Autodesk Inventor part; units mm, degrees
ref_plane "plane_support" through (-5.5, -8, -3) normal (0, -1, 0) x (1, 0, 0)
ref_plane "YZ Plane" through (0, 0, 0) normal (1, 0, 0) x (0, 1, 0)
ref_plane "XZ Plane" through (0, 0, 0) normal (0, 1, 0) x (-1, 0, 0)
sketch "Sketch14" plane through (0, 0, 0) normal (1, 0, 0) x (0, 1, 0)
  line L0 (-13.2, 0) -> (16.2, 0)
  line L1 (0, -4.2) -> (0, 4.2)
  line L2 (9, -3) -> (-9, -3)
  line L3 (-9, -3) -> (-9, 3)
  line L4 (-9, 3) -> (9, 3)
  line L5 (9, 3) -> (9, -3) construction
  line L6 (9, -3) -> (-9, 3) construction
  line L7 (-9, -3) -> (9, 3) construction
  line L8 (5.5, 3) -> (5.5, -3) construction
  line L9 (-6.5, 3) -> (-6.5, -3) construction
  arc A0 (9, -3) -> (9, 3) centre (9, 0) ccw
  circle A1 centre (9, 0) radius 1.25
  circle A2 centre (9, 0) radius 3 construction
  line L10 (6, 3) -> (6, -3) construction
  line L11 (12, -3) -> (9, -3)
  line L12 (9, -3) -> (9, 3)
  line L13 (9, 3) -> (12, 3)
  line L14 (12, 3) -> (12, -3)
  line L15 (12, -3) -> (9, 3) construction
  line L16 (9, -3) -> (12, 3) construction
  point P0 (0, 0)
  point P1 (0, 0)
  point P2 (10.5, 0)
  dimension "d72" = 6
  dimension "d73" = 12
  dimension "d74" = 2.5
  dimension "d75" = 2.5
  dimension "d76" = 0.5
extrude "ext_main" add sketch "Sketch14" along normal mid plane 11
sketch "sk_channel_nut" plane through (-5.5, -9, -3) normal (0, -1, 0) x (1, 0, 0)
  line L0 (-2.2, 3) -> (13.2, 3)
  line L1 (5.5, -1.8497) -> (5.5, 7.8497)
  circle A0 centre (5.5, 3) radius 2
  line L2 (5.5, 6.4641) -> (2.5, 4.7321)
  line L3 (2.5, 4.7321) -> (2.5, 1.2679)
  line L4 (2.5, 1.2679) -> (5.5, -0.4641)
  line L5 (5.5, -0.4641) -> (8.5, 1.2679)
  line L6 (8.5, 1.2679) -> (8.5, 4.7321)
  line L7 (8.5, 4.7321) -> (5.5, 6.4641)
  circle A1 centre (1.5, 3) radius 1
  circle A2 centre (9.5, 3) radius 1
  line L8 (1.5, 4) -> (2.5, 4)
  line L9 (1.5, 2) -> (2.5, 2)
  line L10 (9.5, 4) -> (8.5, 4)
  line L11 (9.5, 2) -> (8.5, 2)
  line L12 (11, 0) -> (0, 0)
  line L13 (11, 6) -> (0, 6)
  line L14 (0, 0) -> (0, 6)
  line L15 (3.4, 6) -> (3.4, 5.2517)
  line L16 (3.4456, 0.722) -> (3.4456, 0)
  line L17 (7.5544, 0.722) -> (7.5544, 0)
  line L18 (7.6, 6) -> (7.6, 5.2517)
  point P0 (5.5, 3)
  point P1 (2.5, 3)
  dimension "d85" = 4
  dimension "d86" = 120
  dimension "d87" = 6
  dimension "d88" = 2
  dimension "d95" = 4.2
extrude "ext_cut_bottomscrews" cut sketch "sk_channel_nut" against normal blind 8 contours A2 L0 | A2 L11 L6 | L6 L10 A2 | L0 A2
extrude "ext_cut_bottom_nut" cut sketch "sk_channel_nut" against normal blind 2 contours L3 L2 L13 L1 A0 L0 | L0 A0 L1 L12 L4 L3 | L16 L4 L12 | L13 L2 L15 | A0 L1 L0 | L0 L1 A0 | L12 L1 L4 | L2 L1 L13 | L1 A0 L0 | L0 A0 L1 | L1 L13 L7 L6 L0 A0 | A0 L0 L6 L5 L12 L1 | L1 L12 L5 | L7 L13 L1 | L5 L17 L12 | L13 L18 L7
sketch "Sketch21" plane through (-5.5, 12, 3) normal (0, 0, 1) x (1, 0, 0)
  line L0 (11, 0) -> (11, -21)
  line L1 (0, 0) -> (11, 0)
  line L2 (0, -21) -> (0, 0)
  line L3 (3.4, -19) -> (7.6, -19)
  line L4 (5.5, 0) -> (5.5, -2.5815) construction
  arc A0 (2, 0) -> (0, -2) centre (2, -2) ccw
  arc A1 (11, -2) -> (9, 0) centre (9, -2) ccw
  circle A2 centre (5.5, -2.5) radius 1.25
  point P0 (5.5, -12)
  point P1 (5.5, -1.25)
  dimension "d106" = 2.5
  dimension "d105" = 2
  dimension "d107" = 1.25
extrude "ext_cut_fronthole" cut sketch "Sketch21" against normal through all
extrude "ext_cut_channel" cut sketch "sk_channel_nut" against normal blind 16 contours A0 L1 L0 | L0 L1 A0 | L1 A0 L0 | L0 A0 L1
extrude "ext_cut_shortscrew" cut sketch "sk_channel_nut" against normal blind 4 contours A1 L0 | L0 A1 | A1 L8 L3 | L3 L9 A1
sketch "Sketch22" plane through (-2.1, -7, 3) normal (0, 0, 1) x (1, 0, 0)
  line L0 (-3.4, -2) -> (-3.4, 17)
  line L1 (0, -2) -> (-3.4, -2)
  line L2 (-3.4, 12) -> (-3.4, 3)
  arc A0 (-3.4, 3) -> (-3.4, 12) centre (-6.2, 7.5) ccw
  line L3 (-3.4, 7.5) -> (-0.9, 7.5) construction
  point P0 (2.1, 7)
  dimension "d112" = 5
  dimension "d113" = 9
  dimension "d119" = 2.5
extrude "ext_cut_cutway" cut sketch "Sketch22" against normal through all
fillet "Fillet1" radius 2 2 edges at (-5.5, 5, 0) (-5.5, -4, 0)
sketch "Sketch19" plane through (-5.5, -8, -3) normal (0, -1, 0) x (1, 0, 0)
  line L0 (3.4, 6) -> (7.6, 6)
  line L1 (3.4, 5.2517) -> (3.4, 6)
  line L2 (2.5, 4.7321) -> (3.4, 5.2517)
  line L3 (2.5, 1.2679) -> (2.5, 2)
  line L4 (3.4456, 0.722) -> (2.5, 1.2679)
  line L5 (3.4456, 0) -> (3.4456, 0.722)
  line L6 (7.5544, 0) -> (3.4456, 0)
  line L7 (7.5544, 0.722) -> (7.5544, 0)
  line L8 (8.5, 1.2679) -> (7.5544, 0.722)
  line L9 (8.5, 2) -> (8.5, 1.2679)
  line L10 (8.5, 4) -> (8.5, 2)
  line L11 (8.5, 4.7321) -> (8.5, 4)
  line L12 (7.6, 5.2517) -> (8.5, 4.7321)
  line L13 (7.6, 6) -> (7.6, 5.2517)
  circle A0 centre (5.5, 3) radius 2
  line L14 (3.8, 5.675) -> (7.275, 5.675) construction
  line L15 (7.275, 5.675) -> (7.275, 5.064)
  line L16 (7.275, 5.064) -> (8.175, 4.5444)
  line L17 (8.175, 4.5444) -> (8.175, 4)
  line L18 (8.175, 4) -> (8.175, 2)
  line L19 (8.175, 2) -> (8.175, 1.4556)
  line L20 (8.175, 1.4556) -> (7.2294, 0.9097)
  line L21 (7.2294, 0.9097) -> (7.2294, 0.325)
  line L22 (7.2294, 0.325) -> (3.7706, 0.325) construction
  line L23 (3.7706, 0.325) -> (3.7706, 0.9097)
  line L24 (3.7706, 0.9097) -> (2.9, 1.4123)
  line L25 (2.9, 1.4123) -> (2.9, 2)
  line L26 (2.9, 2) -> (2.9, 4)
  line L27 (2.9, 4) -> (2.9, 4.5011)
  line L28 (2.9, 4.5011) -> (3.8, 5.0207)
  line L29 (3.8, 5.0207) -> (3.8, 5.675)
  line L30 (3.8, 5.675) -> (7.275, 5.675)
  line L31 (7.275, 5.675) -> (7.275, 6)
  line L32 (7.275, 6) -> (3.8, 6)
  line L33 (3.8, 6) -> (3.8, 5.675)
  line L34 (3.7706, 0.325) -> (7.2294, 0.325)
  line L35 (7.2294, 0.325) -> (7.2294, 0)
  line L36 (7.2294, 0) -> (3.7706, 0)
  line L37 (3.7706, 0) -> (3.7706, 0.325)
  line L38 (2.5, 2) -> (2.5, 4)
  line L39 (2.5, 4) -> (2.5, 4.7321)
  point P0 (5.5, 3)
  dimension "d97" = 0.4
equation "\"d73\" = linact_rod_effective_length"
equation "\"d74\" = nut_m3_thickness_max"
equation "\"d75\" = screw_m2_bore_loose"
equation "\"d87\" = nut_m3_width_acrossflats"
equation "\"d88\" = screw_m2_bore_selfthreading"
equation "\"d95\" = 0.7 * nut_m3_width_acrossflats"
equation "\"d93\" = 0.8 * nut_m3_thickness_max"
equation "\"d106\" = screw_m2_bore_loose"
equation "\"d97\" = print_support_z_clearance"
equation "\"d96\" = print_support_xy_clearance"
properties part number "empty"
Source: CAD feature listing. Evaluate the final solid. Frame: model axes, mm. A direction names the side the tool comes from. Coordinates: 2 decimals unless noted, no trailing zeros. Order: outer loops, then holes, each group sorted by start corner. A loop starts at its lowest first (then second) coordinate and runs counter-clockwise, first axis right, second up. Notation, with made-up numbers: M -29,26 L -2,26 A4 ccw -2,32 Z; hole C 13.25,65.25 d6. An arc over 180 degrees is marked long. Write each question's results on one line, items separated by ' | '. Start each with the question number.
1) Section query B-B (x = 0). Return the cut outline in (y, z), plus the area to 3 significant figures.
2) Section query A-A (y = 9.5). Return the cut outline in (x, z), plus the area to 3 significant figures.
3) Section query C-C (z = 0). Return the cut outline in (x, y), plus the area to 3 significant figures.
4) Section query D-D (y = 5.5). Return the cut outline in (x, z).
5) Line query: line 1 (X direction, y = -6, z = 0.05); line 2 (Y direction, x = 0, z = -1); line 3 (Z direction, x = 0, y = 3). Output: solid intervals per line, ascending. Write a range as from..to.
6) Draft query along Y for faces 4 (the face through (-2.544, -8.014, 1.996)), 5 (the face through (-0.16, 10.74, 0.04)), 6 (the face through (-4, -5, 0)). Return one class per face: released by +Y, released by -Y, zero draft, split by the parting line, or undercut.
7) Contact query for flat-ended pins moving along their axis: pin 1 Ø2.5 at (x, z) = (0, 0) entering from -Y; pin 2 Ø2 at (x, z) = (4.5, 0) entering from -Y. Output: stop coordinate, or through.
8) Access query for faces 1 (the face through (-5.316, 5.162, -0.042)), 2 (the face through (-3.5, -7, 1)), 3 (the face through (5, -9, -1)). Directions: +Z, -Z, +X, -X, +Y, -Y. A direction counts if a zero-diameter tool reaches every point of the face in a straight line with its end or side. Return the directions, or none.
Answers:
1) outline: M -7,-3 L 8.25,-3 L 8.25,3 L -7,3 L -7,2 L 7,2 L 7,-2 L -7,-2 Z; M 10.75,-3 L 12,-3 L 12,3 L 10.75,3 Z | area: 43.0 mm^2
2) outline: M -5.5,-3 L -1.25,-3 L -1.25,3 L -5.5,3 Z; M 1.25,-3 L 5.5,-3 L 5.5,3 L 1.25,3 Z | area: 51.0 mm^2
3) outline: M -5.5,-9 L -5,-9 L -5,-5 L -3,-5 L -3,-7 L -2,-7 L -2,7 L 2,7 L 2,-7 L 3,-7 L 3,-1 L 5,-1 L 5,-9 L 5.5,-9 L 5.5,10 A2 ccw 3.5,12 L -3.5,12 A2 ccw -5.5,10 L -5.5,6 A2 ccw -4.82,4.49 A5.3 cw -4.82,-3.49 A2 ccw -5.5,-5 Z; hole C 0,9.5 d2.5 | area: 116 mm^2
4) outline: M -5.44,-3 L 5.5,-3 L 5.5,3 L -5.44,3 Z; hole C 0,0 d4
5) line 1: x = -5.5..-5, -3..-2, 2..3, 5..5.5 | line 2: y = 7..8.25, 10.75..12 | line 3: z = -3..-2, 2..3
6) face 4: zero draft | face 5: undercut | face 6: released by -Y
7) pin 1: stops at y = 7 | pin 2: stops at y = -9
8) face 1: +Z, -Z, -X | face 2: -Y | face 3: +Z, -Z, +X, -X, -Y
